Work out the finished part from the listing and answer in its coordinate system (mm). A direction names the side the tool comes from. Give positions to 0.01 mm unless a question says otherwise; leave off trailing zeros. Loops run counter-clockwise (first coordinate to the right, second up) from the corner with the lowest first, then second, coordinate; pieces in that order, holes last. Notation, with made-up numbers: M 47.5,11.25 L 82.5,11.25 A26 cw 82.5,29.25 Z; hole C 78.25,52 d9. An arc over 180 degrees is marked long. Use a Markdown table: item, result.
```python
from build123d import *

# Parameters (mm, degrees)
F0_W     = 20
F0_H     = 10
F0_R     = 1.25
F1_DEPTH = 3.225
F3_DEPTH = 2.05
F4_W     = 0.5
F4_H     = 4
F5_DEPTH = 1.75
F6_R     = 0.5
F7_DEPTH = 19.251


with BuildPart() as f1:
    # F0 (on Front) → F1 (new body, symmetric)
    with BuildSketch(Plane.XZ):
        with Locations((0, 5)):
            Rectangle(F0_W, F0_H)
        with Locations((-5, 3)):
            Circle(F0_R, mode=Mode.SUBTRACT)
        with Locations((5, 3)):
            Circle(F0_R, mode=Mode.SUBTRACT)
    extrude(amount=F1_DEPTH, both=True)

    # F2 (on Front) → F3 (join, symmetric)
    with BuildSketch(Plane.XZ):
        Polygon((8.4548132206, 14.1411047216), (-7, 10), (-6.8705904774, 9.5170370869), (8.5842227432, 13.6581418085), align=None)
    extrude(amount=F3_DEPTH, both=True)

    # F4 (on Front) → F5 (join, symmetric)
    with BuildSketch(Plane.XZ):
        with Locations((-9, -2)):
            Rectangle(F4_W, F4_H)
        with Locations((0.5, -2)):
            Rectangle(F4_W, F4_H)
        with Locations((9, -2)):
            Rectangle(F4_W, F4_H)
    extrude(amount=F5_DEPTH, both=True)

    # F6 (on face) → F7 (cut, through all)
    with BuildSketch(Plane(origin=(-9.25, 0, 0), x_dir=(0, -1, 0), z_dir=(-1, 0, 0))):
        with Locations((0, -3)):
            Circle(F6_R)
    extrude(amount=-F7_DEPTH, mode=Mode.SUBTRACT)


solid = f1.part
```
(1) Given P1, Ø4.5, axis at x = 2.5, z = 13, coming from the +Y side; P2, Ø1, axis at y = 0.5, z = -2, coming from the +X side; P3, Ø1.5, axis at x = -5.5, y = -2, coming from the -Z side; P4, Ø1, axis at x = 4.5, z = -2, coming from the +Y side, each flat-ended and moving along its own axis, determine where each tip first touches the part or whether it passes through.
Entries:
| item | result |
|---|---|
| P1 | stops at y = 2.05 |
| P2 | stops at x = 9.25 |
| P3 | stops at z = 0 |
| P4 | passes through |
(2) Which of the six approach directions +Z, -Z, +X, -X, +Y, -Y give full straight-line access (tool end or side, diameter ignored) to faces 1 (the flat face through (1.9, 2.05, 12.1)), 2 (the flat face through (9.25, 0, -2)), 3 (the flat face through (1.662, -0.029, 11.803)), 4 (the flat face through (0.25, 0, -2)), 5 (the flat face through (1.9, -2.05, 12.1))?
Entries:
| item | result |
|---|---|
| face 1 | +Z, +X, -X, +Y |
| face 2 | -Z, +X, +Y, -Y |
| face 3 | +X, +Y, -Y |
| face 4 | -Z, +Y, -Y |
| face 5 | +Z, +X, -X, -Y |
(3) Consider probe 1 along Z at (x, y) = (0.5, 0); probe 2 along Z at (x, y) = (9.05, 0); probe 3 along Z at (x, y) = (5, 1.75). Determine where each line is inside the solid, lowest interval first. Write a range as [from, to].
Entries:
| item | result |
|---|---|
| probe 1 | z = [-4, -3.5], [-2.5, 10], [11.49, 12.01] |
| probe 2 | z = [-4, -3.5], [-2.5, 10] |
| probe 3 | z = [0, 1.75], [4.25, 10], [12.7, 13.22] |
(4) A cutting plane is placed at D-D (z = 3). Write down the section's boundary in (x, y) (3 decimals).
Entries:
| item | result |
|---|---|
| outline | M -10,-3.225 L -6.25,-3.225 L -6.25,3.225 L -10,3.225 Z; M -3.75,-3.225 L 3.75,-3.225 L 3.75,3.225 L -3.75,3.225 Z; M 6.25,-3.225 L 10,-3.225 L 10,3.225 L 6.25,3.225 Z |
(5) A cutting plane is placed at B-B (y = 1.25). Write down the section's boundary in (x, z).
Entries:
| item | result |
|---|---|
| outline | M -10,0 L -9.25,0 L -9.25,-4 L -8.75,-4 L -8.75,0 L 0.25,0 L 0.25,-4 L 0.75,-4 L 0.75,0 L 8.75,0 L 8.75,-4 L 9.25,-4 L 9.25,0 L 10,0 L 10,10 L -5.07,10 L 8.58,13.66 L 8.45,14.14 L -7,10 L -10,10 Z; hole C -5,3 d2.5; hole C 5,3 d2.5 |
(6) A cutting plane is placed at A-A (z = -3). Write down the section's boundary in (x, y).
Entries:
| item | result |
|---|---|
| outline | M -9.25,-1.75 L -8.75,-1.75 L -8.75,-0.5 L -9.25,-0.5 Z; M -9.25,0.5 L -8.75,0.5 L -8.75,1.75 L -9.25,1.75 Z; M 0.25,-1.75 L 0.75,-1.75 L 0.75,-0.5 L 0.25,-0.5 Z; M 0.25,0.5 L 0.75,0.5 L 0.75,1.75 L 0.25,1.75 Z; M 8.75,-1.75 L 9.25,-1.75 L 9.25,-0.5 L 8.75,-0.5 Z; M 8.75,0.5 L 9.25,0.5 L 9.25,1.75 L 8.75,1.75 Z |
(7) The mould has two halves that part along Z. Classify faces 6 (the flat face through (0.84, -0.03, 12.1)), 7 (the cylindrical face through (-9.004, 0.065, -2.504)), 8 (the flat face through (0, -3.225, 5)): released by +Z, released by -Z, zero draft, split by the parting line, or undercut.
Entries:
| item | result |
|---|---|
| face 6 | released by +Z |
| face 7 | undercut |
| face 8 | zero draft |
(8) A cutting plane is placed at C-C (y = 0). Count the separate pieces of the cut face and the enclosed holes in it, and give its area (3 significant figures).
Entries:
| item | result |
|---|---|
| separate pieces | 4 |
| enclosed holes | 2 |
| area | 202 mm² |
